The listing builds one solid part. Answer for the finished solid, in the listing's coordinates (mm). Round coordinates to 2 decimals unless told otherwise and drop trailing zeros. Order: outer loops, then holes, each group sorted by start corner. A loop starts at its lowest first (then second) coordinate and runs counter-clockwise, first axis right, second up. Notation, with made-up numbers: (86, 15.25) - (112, 15.25) arc R18 cw to (112, 26.25) - close; hole circle Ø5 at (-34.5, 16). An arc over 180 degrees is marked (long way). One line per item, written item: value. Start each with the question number.
1. Section B-B, the plane x = 48 is taken. Give the vertices of the cut face in (y, z).
2. Section D-D, the plane y = -2.25 is taken. Give the vertices of the cut face in (x, z).
3. Section A-A, the plane y = -9 is taken. Give the vertices of the cut face in (x, z).
4. Flat-ended cylindrical pins translate along their axes: P1, Ø1, axis at y = -7.5, z = -2, coming from the +X side; P2, Ø1, axis at y = -2.5, z = 1, coming from the -X side; P3, Ø2.5, axis at x = 42.5, z = -0.5, coming from the -Y side. Find the tip coordinate at first contact, or state that the pin passes through.
5. Straight lines are drawn through the part: line 1 (Y direction, x = 36, z = -2.2); line 2 (X direction, y = -6.75, z = -1.45); line 3 (X direction, y = -5.5, z = 2.05). For each, find the intervals that lie inside material, in ascending order.
6. Section C-C, the plane z = 0.5 is taken. Give the vertices of the cut face in (x, y), then the cut area to 3 significant figures.
from build123d import *

# Parameters (mm, degrees)
F1_DEPTH = 10
F2_DEPTH = 5


with BuildPart() as f1:
    # F0 (on Front) → F1 (new body)
    with BuildSketch(Plane.XZ):
        with BuildLine():
            ThreePointArc((0, -2.5), (1.767767, -1.767767), (2.5, 0))
            ThreePointArc((2.5, 0), (1.767767, 1.767767), (0, 2.5))
            Line((0, 2.5), (0, -2.5))
        make_face()
        with BuildLine():
            ThreePointArc((30.5, 0), (29.767767, 1.767767), (28, 2.5))
            ThreePointArc((28, 2.5), (25.5, 0), (28, -2.5))
            ThreePointArc((28, -2.5), (29.767767, -1.767767), (30.5, 0))
        make_face()
        with BuildLine():
            ThreePointArc((54.5, 0), (53.767767, 1.767767), (52, 2.5))
            Line((52, 2.5), (52, -2.5))
            ThreePointArc((52, -2.5), (53.767767, -1.767767), (54.5, 0))
        make_face()
        with BuildLine():
            Line((52, -2.5), (52, 2.5))
            ThreePointArc((52, 2.5), (49.5, 0), (52, -2.5))
        make_face()
        with BuildLine():
            Line((0, -2.5), (0, 2.5))
            ThreePointArc((0, 2.5), (-2.5, 0), (0, -2.5))
        make_face()
    extrude(amount=F1_DEPTH)

    # F0 (on Front) → F2 (join)
    with BuildSketch(Plane.XZ):
        with BuildLine():
            ThreePointArc((0, 2.5), (1.767767, 1.767767), (2.5, 0))
            ThreePointArc((2.5, 0), (1.767767, -1.767767), (0, -2.5))
            Line((0, -2.5), (28, -2.5))
            ThreePointArc((28, -2.5), (25.5, 0), (28, 2.5))
            Line((28, 2.5), (0, 2.5))
        make_face()
        with BuildLine():
            Line((0, -2.5), (0, 2.5))
            ThreePointArc((0, 2.5), (-2.5, 0), (0, -2.5))
        make_face()
        with BuildLine():
            Line((52, 2.5), (28, 2.5))
            ThreePointArc((28, 2.5), (29.767767, 1.767767), (30.5, 0))
            ThreePointArc((30.5, 0), (29.767767, -1.767767), (28, -2.5))
            Line((28, -2.5), (52, -2.5))
            ThreePointArc((52, -2.5), (49.5, 0), (52, 2.5))
        make_face()
        with BuildLine():
            ThreePointArc((54.5, 0), (53.767767, 1.767767), (52, 2.5))
            Line((52, 2.5), (52, -2.5))
            ThreePointArc((52, -2.5), (53.767767, -1.767767), (54.5, 0))
        make_face()
    extrude(amount=F2_DEPTH)


solid = f1.part
Answer list:
1. outline: (-5, -2.5) - (0, -2.5) - (0, 2.5) - (-5, 2.5) - close
2. outline: (0, -2.5) - (52, -2.5) arc R2.5 ccw to (52, 2.5) - (0, 2.5) arc R2.5 ccw to start
3. outline: circle Ø5 at (0, 0); circle Ø5 at (28, 0); circle Ø5 at (52, 0)
4. P1: stops at x = 54
4. P2: stops at x = -2.45
4. P3: stops at y = -5
5. line 1: y = -5 to 0
5. line 2: x = -2.04 to 2.04, 25.96 to 30.04, 49.96 to 54.04
5. line 3: x = -1.43 to 1.43, 26.57 to 29.43, 50.57 to 53.43
6. outline: (-2.45, -10) - (2.45, -10) - (2.45, -5) - (25.55, -5) - (25.55, -10) - (30.45, -10) - (30.45, -5) - (49.55, -5) - (49.55, -10) - (54.45, -10) - (54.45, 0) - (-2.45, 0) - close
6. area: 358 mm²
